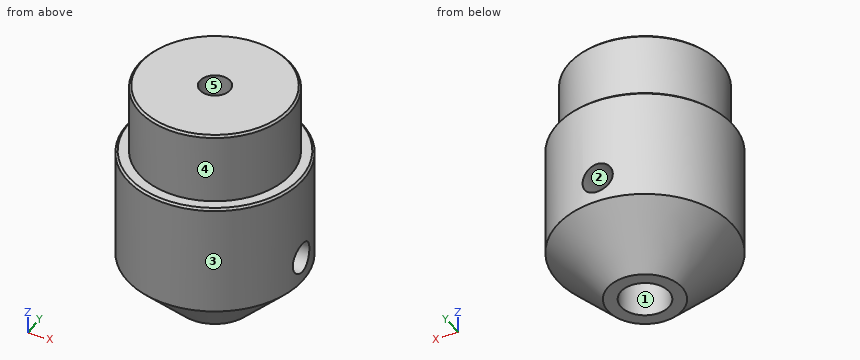
from build123d import *

# Parameters (mm, degrees)
SKETCH1_R                    = 11
BOSS_EXTRUDE1_DEPTH          = 20.32
SKETCH5_R                    = 9.5
BOSS_EXTRUDE6_DEPTH          = 8.89
B_0_238_DIAMETER_HOLE1_D     = 6.0452
B_0_238_DIAMETER_HOLE1_DEPTH = 19.05
B_0_238_DIAMETER_HOLE1_TIP   = 1.816161307
F_10_24_TAPPED_HOLE1_REACH   = 33.504
F_10_24_TAPPED_HOLE1_BORE_R  = 1.89865
F_10_24_TAPPED_HOLE2_D       = 3.7973
CHAMFER1_SIZE                = 6.35
CHAMFER2_SIZE                = 0.254
CIRPATTERN1_COUNT            = 2
CIRPATTERN1_ANGLE            = 90


with BuildPart() as part:
    # Sketch1 → Boss-Extrude1 (new body)
    with BuildSketch(Plane.XY):
        Circle(SKETCH1_R)
    extrude(amount=BOSS_EXTRUDE1_DEPTH)

    # Sketch5 → Boss-Extrude6 (add)
    with BuildSketch(Plane.XY.offset(20.32)):
        Circle(SKETCH5_R)
    extrude(amount=BOSS_EXTRUDE6_DEPTH)

    # B (0.238) Diameter Hole1
    with Locations(Plane(origin=(0, 0, 0), x_dir=(-1, 0, 0), z_dir=(0, 0, -1))):
        with Locations((0, 0)):
            Hole(B_0_238_DIAMETER_HOLE1_D / 2, depth=B_0_238_DIAMETER_HOLE1_DEPTH)
            with Locations((0, 0, -(B_0_238_DIAMETER_HOLE1_DEPTH + B_0_238_DIAMETER_HOLE1_TIP / 2))):  # 118° drill point
                Cone(0, B_0_238_DIAMETER_HOLE1_D / 2, B_0_238_DIAMETER_HOLE1_TIP, mode=Mode.SUBTRACT)

    # #10-24 Tapped Hole1 bore (on position points) → #10-24 Tapped Hole1 (cut, up to next)
    with BuildSketch(Plane(origin=(0, 11, 9.525), x_dir=(1, 0, 0), z_dir=(0, 1, 0)), mode=Mode.PRIVATE) as f_10_24_tapped_hole1_sk1:
        Circle(F_10_24_TAPPED_HOLE1_BORE_R)
    f_10_24_tapped_hole1_tool1 = extrude(f_10_24_tapped_hole1_sk1.sketch, amount=-F_10_24_TAPPED_HOLE1_REACH, mode=Mode.PRIVATE) & part.part
    f_10_24_tapped_hole1 = f_10_24_tapped_hole1_tool1.solids().sort_by_distance((0, 11, 9.525))[0]
    add(f_10_24_tapped_hole1, mode=Mode.SUBTRACT)

    # #10-24 Tapped Hole2 (through all)
    with Locations(Plane.XY.offset(29.21)):
        with Locations((0, 0)):
            Hole(F_10_24_TAPPED_HOLE2_D / 2)

    # Chamfer1
    chamfer1_edges = [part.edges().sort_by_distance(p)[0] for p in [
        (-11, 0, 0),
    ]]
    chamfer(chamfer1_edges, length=CHAMFER1_SIZE)

    # Chamfer2
    chamfer2_edges = [part.edges().sort_by_distance(p)[0] for p in [
        (-11, 0, 20.32),
        (-9.5, 0, 29.21),
    ]]
    chamfer(chamfer2_edges, length=CHAMFER2_SIZE)

    # CirPattern1: #10-24 Tapped Hole1 ×2 about axis
    cirpattern1_axis = Axis((0, 0, 20.32), (0, 0, -1))
    for i in range(1, CIRPATTERN1_COUNT):
        add(f_10_24_tapped_hole1.rotate(cirpattern1_axis, i * CIRPATTERN1_ANGLE / (CIRPATTERN1_COUNT - 1)), mode=Mode.SUBTRACT)


solid = part.part
CAD build for the part. Positions are in the model's coordinates, mm. Face numbers are marked on the shaded views. A direction names the side the tool comes from. Round coordinates to 2 decimals unless told otherwise and drop trailing zeros. Write each loop counter-clockwise with the first axis right and the second up, starting at its lowest first coordinate (ties: lowest second). Pieces come first, ordered by that corner, then holes.
(1) Mould opens along Y. For the marked faces 1, 2 and 3 say: pulls with the +Y half, pulls with the -Y half, needs draft (parallel to the pull), parting line crosses it, or undercut.
(2) Slice it at A-A, the plane x = 0. Write the cut outline in (y, z), and give its area (3 significant figures).
(3) Slice it at C-C, the plane z = 18.5. Write the cut outline in (x, y).
(4) 3-axis set-ups, long thin cutter, end or side, ignore diameter. For the marked faces 4 and 5: which of +Z, -Z, +X, -X, +Y, -Y reach the whole face in a straight line?
(5) Probe line 1 along Y through (x, z) = (0, 22); line 2 along Y through (x, z) = (0, 12.25); line 3 along X through (y, z) = (-0.75, 24). List the from-to ranges inside material, lowest first.
(6) Drop flat-ended pins along their axis: P1, Ø4, axis at y = 3, z = 17, coming from the +X side; P2, Ø3, axis at y = 8.5, z = 18.5, coming from the -X side; P3, Ø10, axis at x = -8.5, z = 3, coming from the -Y side. Give the stop position or say it passes through.
From the geometry:
1. face 1: undercut
1. face 2: needs draft
1. face 3: parting line crosses it
2. outline: (-11, 6.35) - (-4.65, 0) - (-3.02, 0) - (-3.02, 19.05) - (-1.9, 19.73) - (-1.9, 29.21) - (-9.25, 29.21) - (-9.5, 28.96) - (-9.5, 20.32) - (-10.75, 20.32) - (-11, 20.07) - close; (1.9, 19.73) - (3.02, 19.05) - (3.02, 11.42) - (11, 11.42) - (11, 20.07) - (10.75, 20.32) - (9.5, 20.32) - (9.5, 28.96) - (9.25, 29.21) - (1.9, 29.21) - close; (3.02, 0) - (4.65, 0) - (11, 6.35) - (11, 7.63) - (3.02, 7.63) - close
2. area: 391 mm2
3. outline: circle Ø22 at (0, 0); hole circle Ø6.05 at (0, 0)
4. face 4: +Z
4. face 5: +Z, -Z
5. line 1: y = -9.5 to -1.9, 1.9 to 9.5
5. line 2: y = -11 to -3.02, 3.02 to 11
5. line 3: x = -9.47 to -1.74, 1.74 to 9.47
6. P1: stops at x = 10.95
6. P2: stops at x = -8.49
6. P3: stops at y = -9.9
